Study the drawing (mm; zero at the part's minimum x, y, z) and answer. Give positions to 0.01 mm unless a question says otherwise; leave off trailing zeros. Order: outer loops, then holes, each group sorted by start corner. A loop starts at its lowest first (then second) coordinate and runs counter-clockwise, first axis right, second up.
Item 1: Find the intervals of material crossed by line 1 along X through (y, z) = (109.5, 80); line 2 along Z through (x, y) = (146, 127); line 3 along Z through (x, y) = (220, 157), in increasing order.
Item 2: The mould has two halves that part along X. Classify the marked faces 1, 2, 3 and 4: +X half, -X half, draft (parallel to the pull), parting line (faces both ways), or undercut.
Item 3: Given pin 1 Ø20.5 at (y, z) = (127, 88.9) entering from -X; pin 2 Ø10 at (x, z) = (147.5, 73.5) entering from +Y; pin 3 Ø1.5 at (y, z) = (102, 61.5) entering from +X; pin 4 Ø4 at (y, z) = (40, 40.5) entering from +X, each flat-ended and moving along its own axis, determine where each tip first touches the part or whether it passes through.
Item 4: A cutting plane is placed at C-C (x = 127). Write down the section's boundary in (y, z).
Item 5: A cutting plane is placed at D-D (z = 21). Write down the section's boundary in (x, y), plus the area to 3 significant figures.
Item 6: A cutting plane is placed at A-A (y = 127). Write down the section's boundary in (x, z).
Item 7: A cutting plane is placed at B-B (z = 61). Write down the section's boundary in (x, y).
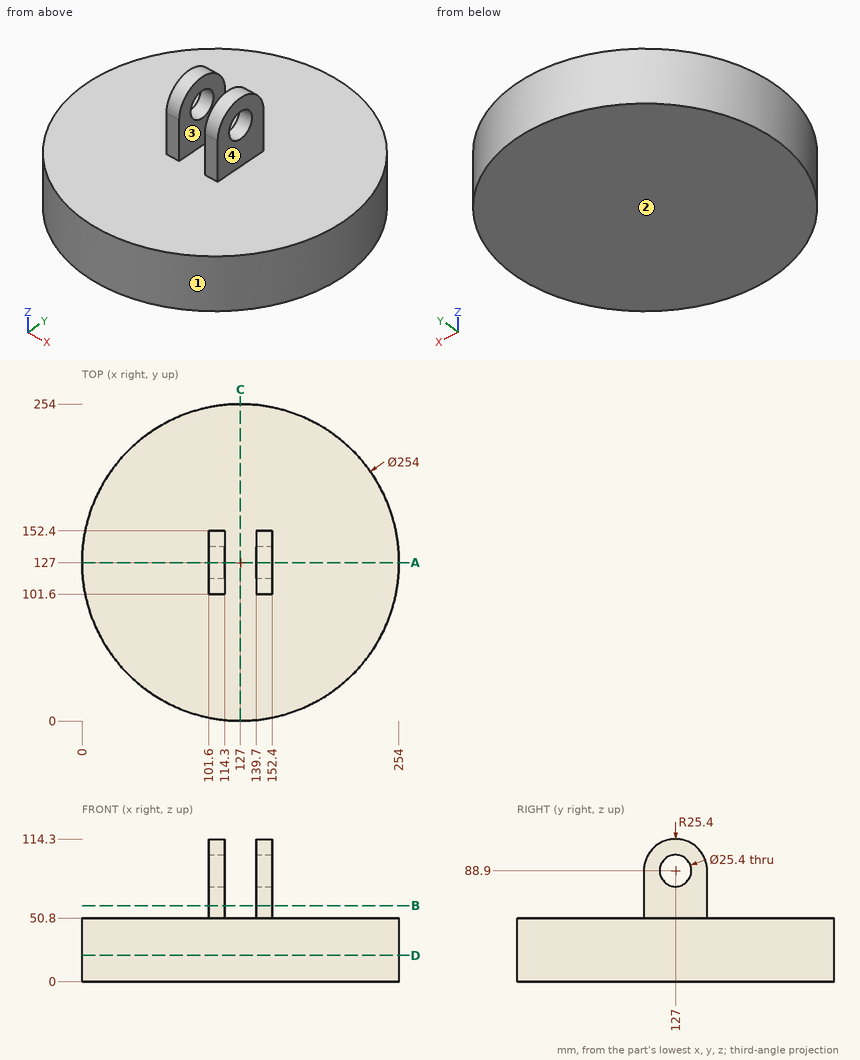
Response values:
1. line 1: x = 101.6 to 114.3, 139.7 to 152.4
1. line 2: z = 0 to 76.2, 101.6 to 114.3
1. line 3: z = 0 to 50.8
2. face 1: parting line
2. face 2: draft
2. face 3: undercut
2. face 4: +X half
3. pin 1: passes through
3. pin 2: stops at y = 152.4
3. pin 3: stops at x = 152.4
3. pin 4: stops at x = 221.36
4. outline: (0, 0) - (254, 0) - (254, 50.8) - (0, 50.8) - close
5. outline: circle Ø254 at (127, 127)
5. area: 50,700 mm2
6. outline: (0, 0) - (254, 0) - (254, 50.8) - (152.4, 50.8) - (152.4, 76.2) - (139.7, 76.2) - (139.7, 50.8) - (114.3, 50.8) - (114.3, 76.2) - (101.6, 76.2) - (101.6, 50.8) - (0, 50.8) - close; (101.6, 101.6) - (114.3, 101.6) - (114.3, 114.3) - (101.6, 114.3) - close; (139.7, 101.6) - (152.4, 101.6) - (152.4, 114.3) - (139.7, 114.3) - close
7. outline: (101.6, 101.6) - (114.3, 101.6) - (114.3, 152.4) - (101.6, 152.4) - close; (139.7, 101.6) - (152.4, 101.6) - (152.4, 152.4) - (139.7, 152.4) - close
